```python
from build123d import *

# Parameters (mm, degrees)
F0_W     = 1
F0_H     = 24
F0_H_2   = 1
F0_W_2   = 24
F1_DEPTH = 150
F2_R     = 3.15
F3_DEPTH = 1


with BuildPart() as f1:
    # F0 (on Right) → F1 (new body)
    with BuildSketch(Plane.YZ):
        with Locations((-4.966528, 10.346573)):
            Rectangle(F0_W, F0_H)
        with Locations((-4.966528, 22.846573)):
            Rectangle(F0_W, F0_H_2)
        with Locations((7.533472, 22.846573)):
            Rectangle(F0_W_2, F0_H_2)
    extrude(amount=F1_DEPTH)

    # F2 (on face) → F3 (cut)
    with BuildSketch(Plane.XY.offset(23.346573)):
        with Locations((15, 3.033472)):
            Circle(F2_R)
        with Locations((45, 3.033472)):
            Circle(F2_R)
        with Locations((75, 3.033472)):
            Circle(F2_R)
        with Locations((105, 3.033472)):
            Circle(F2_R)
        with Locations((135, 3.033472)):
            Circle(F2_R)
    extrude(amount=-F3_DEPTH, mode=Mode.SUBTRACT)


solid = f1.part
```
CAD build for the part. Positions are in the model's coordinates, mm. A direction names the side the tool comes from. Coordinates: 2 decimals unless noted, no trailing zeros. Order: outer loops, then holes, each group sorted by start corner. A loop starts at its lowest first (then second) coordinate and runs counter-clockwise, first axis right, second up. Notation, with made-up numbers: (-31, 66.25) - (2, 66.25) arc R32 cw to (2, 102.25) - close; hole circle Ø6 at (-23.5, 4.5). An arc over 180 degrees is marked (long way). Use a Markdown table: item, result. Add a question column.
(1) Flat gauge pins, fed straight in: pin 1 (3 mm diameter, centred on x = 121, z = 18, fed in from +Y); pin 2 (7 mm diameter, centred on x = 45, y = 3.03, fed in from -Z); pin 3 (5 mm diameter, centred on x = 135, y = 3.03, fed in from +Z). Where does each tip first touch, or does it go through?
(2) Saw through at D-D (x = 15.5). Give the cut face in (y, z), then the cut area to 3 significant figures.
(3) Saw through at A-A (x = 75). Give the cut face in (y, z).
(4) Saw through at C-C (z = 15.75). Give the cut face in (x, y).
(5) Pull direction X, two halves, no side cores. Call faces 3 (the face through (150, 1, 23)), 4 (the face through (11.853, 3.172, 22.854)), 5 (the face through (74, -5.467, 11)): +X half, -X half, draft (parallel to the pull), parting line (faces both ways), or undercut.
(6) Drill centre lines: line 1 along Y through (x, z) = (75, 22.95); line 2 along Z through (x, y) = (120, 16.5); line 3 along Y through (x, z) = (139.5, 9.5). Where is each one in solid material? Low to high. Write a range as [from, to].
(7) Saw through at B-B (y = 17). Give the cut face in (x, z), then the cut area to 3 significant figures.
(8) Which spindle directions (+Z, -Z, +X, -X, +Y, -Y) get a long thin tool onto all of the face, cutting with end or side? Do faces 1 (the face through (74, -4.467, 10)), 2 (the face through (71.853, 3.172, 22.854)). Say none if no direction does.
Solved:
| question | item | result |
|---|---|---|
| 1 | pin 1 | stops at y = -4.47 |
| 1 | pin 2 | stops at z = 22.35 |
| 1 | pin 3 | passes through |
| 2 | outline | (-5.47, -1.65) - (-4.47, -1.65) - (-4.47, 22.35) - (-0.08, 22.35) - (-0.08, 23.35) - (-5.47, 23.35) - close; (6.14, 22.35) - (19.53, 22.35) - (19.53, 23.35) - (6.14, 23.35) - close |
| 2 | area | 42.8 mm² |
| 3 | outline | (-5.47, -1.65) - (-4.47, -1.65) - (-4.47, 22.35) - (-0.12, 22.35) - (-0.12, 23.35) - (-5.47, 23.35) - close; (6.18, 22.35) - (19.53, 22.35) - (19.53, 23.35) - (6.18, 23.35) - close |
| 4 | outline | (0, -5.47) - (150, -5.47) - (150, -4.47) - (0, -4.47) - close |
| 5 | face 3 | +X half |
| 5 | face 4 | undercut |
| 5 | face 5 | draft |
| 6 | line 1 | y = [-5.47, -0.12], [6.18, 19.53] |
| 6 | line 2 | z = [22.35, 23.35] |
| 6 | line 3 | y = [-5.47, -4.47] |
| 7 | outline | (0, 22.35) - (150, 22.35) - (150, 23.35) - (0, 23.35) - close |
| 7 | area | 150 mm² |
| 8 | face 1 | -Z, +X, -X, +Y |
| 8 | face 2 | +Z, -Z |
